Check sheet for the modelled part. Datum: model origin and axes. Units: mm. A direction names the side the tool comes from. Round coordinates to 2 decimals unless told otherwise and drop trailing zeros. Loops run counter-clockwise (first coordinate to the right, second up) from the corner with the lowest first, then second, coordinate; pieces in that order, holes last. Notation, with made-up numbers: (-0.75, 1) - (34.25, 1) arc R20 ccw to (34.25, 12) - close; hole circle Ø6 at (28.25, 20.25). An arc over 180 degrees is marked (long way). Answer in a Markdown table with one row per item. Add a question column.
(1) Cross-section at A-A on x = 19.5. Enter the section's corners in (y, z), then the cut area to 3 significant figures.
(2) Cross-section at B-B on z = 5.5. Enter the section's corners in (x, y), then the cut area to 3 significant figures.
(3) Mould release check, pull along Z, two halves, no side actions. Record for faces 3 (the flat face through (-1.42, -3.92, 7)), 4 (the flat face through (14.508, 8.276, -1.972)), 5 (the flat face through (6, 0, -4)): +Z half, -Z half, draft (parallel to the pull), parting line (faces both ways), or undercut.
(4) Access from +Z, -Z, +X, -X, +Y, -Y to the whole of each face (thin tool, end or side, straight path). Record for faces 1 (the flat face through (7, -11, 0)), 2 (the cylindrical face through (-5.84, 12.95, -1.97)).
(5) Cross-section at C-C on y = 9.75. Enter the section's corners in (x, z), then the cut area to 3 significant figures.
(6) Thickness scan on line 1 along Y through (x, z) = (0, 3.9); line 2 along Y through (x, z) = (-18.5, -1.25); line 3 along Y through (x, z) = (0, -1). Record the ranges inside material, lowest first.
(7) Gauge pin test, flat ends, axial feed: pin 1 (3 mm diameter, centred on x = -7, y = 3.5, fed in from +Z); pin 2 (2 mm diameter, centred on x = -7, z = -1.5, fed in from -Y); pin 3 (4 mm diameter, centred on y = 2.5, z = 4.5, fed in from -X). Record the tip position at first contact, or that the pin passes through.
(8) Cross-section at D-D on x = -18.5. Enter the section's corners in (y, z).
from build123d import *

# Parameters (mm, degrees)
SKETCH_R        = 12.85
PAD_DEPTH       = 4
SKETCH003_R     = 11
POCKET_DEPTH    = 0.5
SKETCH004_R     = 6
PAD001_DEPTH    = 3.5
SKETCH006_R     = 1.5
PAD002_DEPTH    = 6.5
SKETCH005_R     = 4
POCKET001_DEPTH = 7.001
SKETCH007_R     = 2.6
PAD003_DEPTH    = 4
SKETCH008_R     = 4
POCKET002_DEPTH = 4


with BuildPart() as part:
    # Sketch → Pad (new body)
    with BuildSketch(Plane.XY):
        Circle(SKETCH_R)
    extrude(amount=PAD_DEPTH)

    # Sketch003 → Pocket (cut)
    with BuildSketch(Plane.XY.offset(4)):
        Circle(SKETCH003_R)
    extrude(amount=-POCKET_DEPTH, mode=Mode.SUBTRACT)

    # Sketch004 (on Face5 of Pocket) → Pad001 (join)
    with BuildSketch(Plane.XY.offset(3.5)):
        Circle(SKETCH004_R)
    extrude(amount=PAD001_DEPTH)

    # Sketch006 → Pad002 (join)
    with BuildSketch(Plane.XZ):
        with Locations((0, 5)):
            Circle(SKETCH006_R)
    extrude(amount=PAD002_DEPTH)

    # Sketch005 (on Face7 of Pad001) → Pocket001 (cut, through all)
    with BuildSketch(Plane.XY.offset(7)):
        Circle(SKETCH005_R)
    extrude(amount=-POCKET001_DEPTH, mode=Mode.SUBTRACT)

    # Sketch007 → Pad003 (join)
    with BuildSketch(Plane.XY):
        with BuildLine():
            Line((-3.542445, 13.25), (4.373404, 13.25))
            ThreePointArc((7.251161, 12.477086), (5.863276, 13.053407), (4.373404, 13.25))
            Line((7.251161, 12.477086), (21.969939, 3.956011))
            ThreePointArc((23.65, 1.04209), (23.1999, 2.72387), (21.969939, 3.956011))
            Line((23.65, 1.04209), (23.65, -1.322208))
            ThreePointArc((21.959502, -4.246432), (23.196964, -3.011059), (23.65, -1.322208))
            Line((8.3652, -12.074699), (21.959502, -4.246432))
            ThreePointArc((3.969015, -13.25), (6.244305, -12.951104), (8.3652, -12.074699))
            Line((3.969015, -13.25), (-2.715889, -13.25))
            ThreePointArc((-8.759411, -11.630643), (-5.844246, -12.838144), (-2.715889, -13.25))
            Line((-21.777636, -4.114568), (-8.759411, -11.630643))
            ThreePointArc((-23.65, -0.871538), (-23.148302, -2.743902), (-21.777636, -4.114568))
            Line((-23.65, -0.871538), (-23.65, 1.686966))
            ThreePointArc((-22.483817, 3.706854), (-23.337522, 2.853149), (-23.65, 1.686966))
            Line((-8.043592, 12.043921), (-22.483817, 3.706854))
            ThreePointArc((-3.542445, 13.25), (-5.87241, 12.943254), (-8.043592, 12.043921))
        make_face()
        with Locations((-18.5, -0.045589)):
            Circle(SKETCH007_R, mode=Mode.SUBTRACT)
        with Locations((19.5, 0)):
            Circle(SKETCH007_R, mode=Mode.SUBTRACT)
    extrude(amount=-PAD003_DEPTH)

    # Sketch008 → Pocket002 (cut)
    with BuildSketch(Plane.XY):
        Circle(SKETCH008_R)
    extrude(amount=-POCKET002_DEPTH, mode=Mode.SUBTRACT)


solid = part.part
Answers:
| question | item | result |
|---|---|---|
| 1 | outline | (-5.66, -4) - (-2.6, -4) - (-2.6, 0) - (-5.66, 0) - close; (2.6, -4) - (5.39, -4) - (5.39, 0) - (2.6, 0) - close |
| 1 | area | 23.4 mm^2 |
| 2 | outline | (-1.41, -6.5) - (1.41, -6.5) - (1.41, -5.83) arc R6 ccw (long way) to (-1.41, -5.83) - close; hole circle Ø8 at (0, 0) |
| 2 | area | 64.4 mm^2 |
| 3 | face 3 | +Z half |
| 3 | face 4 | draft |
| 3 | face 5 | -Z half |
| 4 | face 1 | +Z |
| 4 | face 2 | +Z, -Z, -X, +Y |
| 5 | outline | (-12.02, -4) - (11.96, -4) - (11.96, 0) - (8.37, 0) - (8.37, 4) - (5.09, 4) - (5.09, 3.5) - (-5.09, 3.5) - (-5.09, 4) - (-8.37, 4) - (-8.37, 0) - (-12.02, 0) - close |
| 5 | area | 158 mm^2 |
| 6 | line 1 | y = -12.85 to -11, -6.5 to -4, 4 to 6, 11 to 12.85 |
| 6 | line 2 | y = -6.01 to -2.65, 2.55 to 6.01 |
| 6 | line 3 | y = -13.25 to -4, 4 to 13.25 |
| 7 | pin 1 | stops at z = 3.5 |
| 7 | pin 2 | stops at y = -12.8 |
| 7 | pin 3 | stops at x = -12.84 |
| 8 | outline | (-6.01, -4) - (-2.65, -4) - (-2.65, 0) - (-6.01, 0) - close; (2.55, -4) - (6.01, -4) - (6.01, 0) - (2.55, 0) - close |
